Design review of the part built by this model. Coordinates are the model's own, in mm. A direction names the side the tool comes from. Give positions to 0.01 mm unless a question says otherwise; leave off trailing zeros. Order: outer loops, then holes, each group sorted by start corner. A loop starts at its lowest first (then second) coordinate and runs counter-clockwise, first axis right, second up. Notation, with made-up numbers: (41, 40.25) -> (46, 40.25) arc R36 cw to (46, 76.25) -> close; hole circle Ø7 at (17.5, 62.25). An arc over 180 degrees is marked (long way). Answer in a Markdown table with one row per item. Add a question column.
```python
from build123d import *

# Parameters (mm, degrees)
BOSS_EXTRUDE1_DEPTH = 17
SKETCH3_R           = 3.25
CUT_EXTRUDE1_DEPTH  = 6
SKETCH4_R           = 3
BOSS_EXTRUDE2_DEPTH = 8


with BuildPart() as part:
    # Sketch2 → Boss-Extrude1 (new body)
    with BuildSketch(Plane.XY):
        Polygon((-60.590688259, -20.348178138), (89.409311741, -20.348178138), (89.409311741, -5.348178138), (69.749311741, -5.348178138), (69.749311741, -15.348178138), (34.109311741, -15.348178138), (34.109311741, -5.348178138), (-60.590688259, -5.348178138), align=None)
    extrude(amount=BOSS_EXTRUDE1_DEPTH)

    # Sketch3 → Cut-Extrude1 (cut)
    with BuildSketch(Plane(origin=(0, 0, 0), x_dir=(-1, 0, 0), z_dir=(0, 0, -1))):
        with Locations((-14.409311741, -12.848178138)):
            Circle(SKETCH3_R)
        with Locations((51.590688259, -12.848178138)):
            Circle(SKETCH3_R)
    extrude(amount=-CUT_EXTRUDE1_DEPTH, mode=Mode.SUBTRACT)

    # Sketch4 → Boss-Extrude2 (add)
    with BuildSketch(Plane.XY.offset(17)):
        with Locations(Location((-51.590688259, -12.848178138, 0), (0, 0, 180))):
            Circle(SKETCH4_R)
    extrude(amount=BOSS_EXTRUDE2_DEPTH)


solid = part.part
```
1) Add section C-C, the plane x = -33. Write out the cut boundary in (y, z), and give its area (3 significant figures).
2) Add section D-D, the plane z = 2.75. Write out the cut boundary in (x, y), and give its area (3 significant figures).
3) Mouldability with a two-part tool opening along Y and no side actions: class faces 6 (the face through (-60.591, -13, 8)), 7 (the face through (-13, -5.348, 8)), 8 (the face through (17.656, -12.705, 2.958)) as +Y half, -Y half, draft (parallel to the pull), parting line (faces both ways), or undercut.
4) For L1, parallel to X at y = -12, z = 10.75; L2, parallel to X at y = -14.75, z = 4; L3, parallel to Z at x = 72, y = -14, list the stretches that pass through material, from the lowest coordinate up.
5) Machinability: for faces 1 (the face through (52, -15.348, 8)), 2 (the face through (14, -13, 6)), 3 (the face through (80, -5.348, 8)), 4 (the face through (13, -20.348, 8)), 5 (the face through (-54.362, -11.699, 20.944)), which of the approach directions +Z, -Z, +X, -X, +Y, -Y give a long, thin tool a straight path to every point of the face, cutting with its end or side? Answer none if there is none.
6) Clearance check with flat-ended pins moving along their axes: P1, Ø5, axis at x = 45.5, z = 6, coming from the +Y side; P2, Ø6, axis at x = -51.59, y = -12.85, coming from the -Z side; P3, Ø5, axis at x = 15.5, y = -13, coming from the -Z side; P4, Ø1, axis at y = -10, z = 18.5, coming from the -X side. State where each tip first meets the part, or that it passes through.
7) Add section A-A, the plane y = -7.5. Write out the cut boundary in (x, z).
8) Add section B-B, the plane z = 10.5. Write out the cut boundary in (x, y).
Verdict:
| question | item | result |
|---|---|---|
| 1 | outline | (-20.35, 0) -> (-5.35, 0) -> (-5.35, 17) -> (-20.35, 17) -> close |
| 1 | area | 255 mm2 |
| 2 | outline | (-60.59, -20.35) -> (89.41, -20.35) -> (89.41, -5.35) -> (69.75, -5.35) -> (69.75, -15.35) -> (34.11, -15.35) -> (34.11, -5.35) -> (-60.59, -5.35) -> close; hole circle Ø6.5 at (-51.59, -12.85); hole circle Ø6.5 at (14.41, -12.85) |
| 2 | area | 1,830 mm2 |
| 3 | face 6 | draft |
| 3 | face 7 | +Y half |
| 3 | face 8 | undercut |
| 4 | L1 | x = -60.59 to 34.11, 69.75 to 89.41 |
| 4 | L2 | x = -60.59 to -54.23, -48.96 to 11.77, 17.04 to 34.11, 69.75 to 89.41 |
| 4 | L3 | z = 0 to 17 |
| 5 | face 1 | +Z, -Z, +Y |
| 5 | face 2 | -Z |
| 5 | face 3 | +Z, -Z, +X, -X, +Y |
| 5 | face 4 | +Z, -Z, +X, -X, -Y |
| 5 | face 5 | +Z |
| 6 | P1 | stops at y = -15.35 |
| 6 | P2 | stops at z = 6 |
| 6 | P3 | stops at z = 0 |
| 6 | P4 | stops at x = -53.46 |
| 7 | outline | (-60.59, 0) -> (34.11, 0) -> (34.11, 17) -> (-60.59, 17) -> close; (69.75, 0) -> (89.41, 0) -> (89.41, 17) -> (69.75, 17) -> close |
| 8 | outline | (-60.59, -20.35) -> (89.41, -20.35) -> (89.41, -5.35) -> (69.75, -5.35) -> (69.75, -15.35) -> (34.11, -15.35) -> (34.11, -5.35) -> (-60.59, -5.35) -> close |
